from build123d import *

# Parameters (mm, degrees)
F0_W      = 38.1
F0_H      = 19.05
F1_DEPTH  = 50.8
F3_D      = 9.8044
F4_W      = 50.8
F4_H      = 19.05
F4_H_2    = 38.1
F5_DEPTH  = 12.7
F7_W      = 40.64
F7_H      = 43.18
F8_DEPTH  = 69.85
F9_W      = 40.64
F9_H      = 43.18
F10_DEPTH = 6.35
F12_DEPTH = 9.525
F14_D     = 3.4544
F14_DEPTH = 12.7
F14_TIP   = 1.0378064612
F15_R     = 12.7
F16_R     = 12.7
F17_R     = 4.7625
F19_DEPTH = 25.4
F20_W     = 41.275
F20_H     = 76.2
F21_DEPTH = 2.54


with BuildPart() as f1:
    # F0 (on Right) → F1 (new body)
    with BuildSketch(Plane.YZ):
        Polygon((0, 63.5), (0, 0), (19.05, 0), (57.15, 0), (76.2, 0), (76.2, 63.5), align=None)
        with Locations((38.1, -9.525)):
            Rectangle(F0_W, F0_H)
    extrude(amount=F1_DEPTH)

    # F3 (through all)
    with Locations(Plane(origin=(0, 0, 0), x_dir=(0, -1, 0), z_dir=(-1, 0, 0))):
        with Locations((-38.1, 31.75)):
            Hole(F3_D / 2)

    # F4 (on face) → F5 (join)
    with BuildSketch(Plane(origin=(0, 0, -19.05), x_dir=(1, 0, 0), z_dir=(0, 0, -1))):
        with Locations((25.4, -9.525)):
            Rectangle(F4_W, F4_H)
        with Locations((25.4, -66.675)):
            Rectangle(F4_W, F4_H)
        with Locations((25.4, -38.1)):
            Rectangle(F4_W, F4_H_2)
    extrude(amount=F5_DEPTH)

    # F7 (on face) → F8 (cut)
    with BuildSketch(Plane.XZ):
        with Locations((30.48, 31.75)):
            Rectangle(F7_W, F7_H)
    extrude(amount=-F8_DEPTH, mode=Mode.SUBTRACT)

    # F9 (on face) → F10 (cut)
    with BuildSketch(Plane.XZ):
        with Locations((30.48, 31.75)):
            Rectangle(F9_W, F9_H)
        Polygon((50.8, 53.34), (50.8, 56.515), (6.985, 56.515), (6.985, 6.985), (50.8, 6.985), (50.8, 10.16), (10.16, 10.16), (10.16, 53.34), align=None)
    extrude(amount=-F10_DEPTH, mode=Mode.SUBTRACT)

    # F11 (on face) → F12 (cut)
    with BuildSketch(Plane.YZ.offset(50.8)):
        Polygon((19.05, -19.05), (0, -19.05), (0, -31.75), (76.2, -31.75), (76.2, -19.05), (57.15, -19.05), align=None)
    extrude(amount=-F12_DEPTH, mode=Mode.SUBTRACT)

    # F14
    with Locations(Plane.YZ.offset(50.8)):
        with Locations((12.7, 58.42), (63.5, 58.42), (12.7, 5.08), (63.5, 5.08)):
            Hole(F14_D / 2, depth=F14_DEPTH)
            with Locations((0, 0, -(F14_DEPTH + F14_TIP / 2))):  # 118° drill point
                Cone(0, F14_D / 2, F14_TIP, mode=Mode.SUBTRACT)

    # F15
    f15_edges = [f1.edges().sort_by_distance(p)[0] for p in [
        (30.48, 69.85, 53.34),
    ]]
    fillet(f15_edges, radius=F15_R)

    # F16
    f16_edges = [f1.edges().sort_by_distance(p)[0] for p in [
        (30.48, 69.85, 10.16),
    ]]
    fillet(f16_edges, radius=F16_R)

    # F17
    f17_edges = [f1.edges().sort_by_distance(p)[0] for p in [
        (6.985, 3.175, 56.515),
        (6.985, 3.175, 6.985),
    ]]
    fillet(f17_edges, radius=F17_R)

    # F18 (on face) → F19 (cut)
    with BuildSketch(Plane.XY.offset(63.5)):
        with BuildLine():
            ThreePointArc((25.0825, 15.08125), (26.7662980227, 14.3837980227), (27.46375, 12.7))
            ThreePointArc((27.46375, 12.7), (26.7662980227, 11.0162019773), (25.0825, 10.31875))
            Line((25.0825, 10.31875), (32.7025, 10.31875))
            ThreePointArc((32.7025, 10.31875), (30.32125, 12.7), (32.7025, 15.08125))
            Line((32.7025, 15.08125), (25.0825, 15.08125))
        make_face()
        with BuildLine():
            ThreePointArc((35.08375, 12.7), (34.3862980227, 14.3837980227), (32.7025, 15.08125))
            ThreePointArc((32.7025, 15.08125), (30.32125, 12.7), (32.7025, 10.31875))
            ThreePointArc((32.7025, 10.31875), (34.3862980227, 11.0162019773), (35.08375, 12.7))
        make_face()
        with BuildLine():
            ThreePointArc((25.0825, 10.31875), (26.7662980227, 11.0162019773), (27.46375, 12.7))
            ThreePointArc((27.46375, 12.7), (26.7662980227, 14.3837980227), (25.0825, 15.08125))
            ThreePointArc((25.0825, 15.08125), (22.70125, 12.7), (25.0825, 10.31875))
        make_face()
    extrude(amount=-F19_DEPTH, mode=Mode.SUBTRACT)

    # F20 (on face) → F21 (cut)
    with BuildSketch(Plane(origin=(0, 0, -31.75), x_dir=(1, 0, 0), z_dir=(0, 0, -1))):
        with Locations((20.6375, -38.1)):
            Rectangle(F20_W, F20_H)
    extrude(amount=-F21_DEPTH, mode=Mode.SUBTRACT)


solid = f1.part
Check sheet for the modelled part. Datum: model origin and axes. Units: mm. A direction names the side the tool comes from. Give positions to 0.01 mm unless a question says otherwise; leave off trailing zeros. Order: outer loops, then holes, each group sorted by start corner. A loop starts at its lowest first (then second) coordinate and runs counter-clockwise, first axis right, second up. Notation, with made-up numbers: M 27.25,5.5 L 79.25,5.5 A29 ccw 79.25,28.5 Z; hole C -33,-5.5 d9. An arc over 180 degrees is marked long. Answer as CSV lines item,"result". Start each with the question number.
Item 1: Cross-section at A-A on z = 31.75. Enter the section's corners in (x, y) (3 decimals), plus the area to 3 significant figures.
Item 2: Cross-section at C-C on x = 28. Enter the section's corners in (y, z) (3 decimals), plus the area to 3 significant figures.
Item 3: Cross-section at B-B on y = 38.1. Enter the section's corners in (x, z) (3 decimals).
Item 4: Thickness scan on line 1 (Z direction, x = 45.25, y = 12.7); line 2 (Y direction, x = 41.5, z = 5.08); line 3 (Z direction, x = 31.5, y = 54). Record the ranges inside material, lowest first. Write a range as [from, to].
Item 5: Cross-section at D-D on y = 24. Enter the section's corners in (x, z) (3 decimals).
Item 6: Gauge pin test, flat ends, axial feed: P1, Ø12, axis at x = 31, z = 52.5, coming from the -Y side; P2, Ø5.5, axis at x = 31, z = -7, coming from the -Y side; P3, Ø19.5, axis at x = 20.5, z = 32, coming from the -Y side; P4, Ø3, axis at y = 63.5, z = 5.08, coming from the +X side. Record the tip position at first contact, or that the pin passes through.
Item 7: Tool access check on faces 1 (the face through (30, 69.85, 32)), 2 (the face through (44.361, 63.725, 60.133)), 3 (the face through (20, 9, -19.05)). Record the directions out of +Z, -Z, +X, -X, +Y, -Y that give a thin tool (end or side, any length) a straight path to the whole face; none if there is none.
Item 8: Mould release check, pull along X, two halves, no side actions. Record for faces 4 (the face through (30.76, 66.03, 49.72)), 5 (the face through (22.7, 12.75, 58.49)), 6 (the face through (8.42, 3.22, 55.16)): +X half, -X half, draft (parallel to the pull), parting line (faces both ways), or undercut.
Established:
1,outline,"M 0,0 L 6.985,0 L 6.985,6.35 L 10.16,6.35 L 10.16,33.198 L 0,33.198 Z; M 0,43.002 L 10.16,43.002 L 10.16,69.85 L 50.8,69.85 L 50.8,76.2 L 0,76.2 Z"
1,area,"912 mm^2"
2,outline,"M 0,-29.21 L 76.2,-29.21 L 76.2,-19.05 L 57.15,-19.05 L 57.15,0 L 76.2,0 L 76.2,63.5 L 15.081,63.5 L 15.081,53.34 L 57.15,53.34 A12.7 cw 69.85,40.64 L 69.85,22.86 A12.7 cw 57.15,10.16 L 6.35,10.16 L 6.35,6.985 L 0,6.985 L 0,0 L 19.05,0 L 19.05,-19.05 L 0,-19.05 Z; M 0,56.515 L 6.35,56.515 L 6.35,53.34 L 10.319,53.34 L 10.319,63.5 L 0,63.5 Z"
2,area,"3,300 mm^2"
3,outline,"M 0,-29.21 L 41.275,-29.21 L 41.275,-19.05 L 50.8,-19.05 L 50.8,10.16 L 10.16,10.16 L 10.16,26.848 L 0,26.848 Z; M 0,36.652 L 10.16,36.652 L 10.16,53.34 L 50.8,53.34 L 50.8,63.5 L 0,63.5 Z"
4,line 1,"z = [0, 3.35], [6.81, 10.16], [53.34, 56.69], [60.15, 63.5]"
4,line 2,"y = [0, 10.97], [14.43, 61.77], [65.23, 76.2]"
4,line 3,"z = [-29.21, 10.16], [53.34, 63.5]"
5,outline,"M 0,-29.21 L 41.275,-29.21 L 41.275,-19.05 L 50.8,-19.05 L 50.8,10.16 L 10.16,10.16 L 10.16,53.34 L 50.8,53.34 L 50.8,63.5 L 0,63.5 Z"
6,P1,"stops at y = 0"
6,P2,"stops at y = 19.05"
6,P3,"stops at y = 69.8"
6,P4,"stops at x = 37.96"
7,face 1,"+X, -Y"
7,face 2,"+X"
7,face 3,"+X, -X, -Y"
8,face 4,"draft"
8,face 5,"undercut"
8,face 6,"+X half"
